Input: part model. Units: mm. Frame: model coordinates. Coordinates: 2 decimals unless noted, no trailing zeros. Write each loop counter-clockwise with the first axis right and the second up, starting at its lowest first coordinate (ties: lowest second). Pieces come first, ordered by that corner, then holes. Notation, with made-up numbers: (-35, 62.5) - (-16, 62.5) arc R21 ccw to (-16, 95.5) - close; hole circle Ø4 at (22.25, -7). An arc over 180 degrees is marked (long way). Use a Markdown table: item, result. Add a question column.
Q1. Section query A-A (z = 0). Return the cut outline in (x, y) (1 decimal), then the cut area to 3 significant figures.
Q2. Material intervals for probe 1 along Z at (x, y) = (-28, 0) (1 decimal); probe 2 along X at (y, z) = (-1.25, 6.25), sorted ascending. Write a range as from..to.
Q3. Pin query (flat end, axial travel): P1, Ø8, axis at x = 156.5, z = 3, coming from the -Y side; P2, Ø6, axis at x = -359, z = -6, coming from the +Y side; P3, Ø2, axis at y = -5, z = -5.5, coming from the -X side; P4, Ø2, axis at x = -271, y = -4.5, coming from the +Z side. Return the tip coordinate at first contact, or that it passes through.
from build123d import *

# Parameters (mm, degrees)
SKETCH_1_R        = 7.9375
SKETCH_1_R_2      = 3.975
EXTRUDE_1_DEPTH   = 493.649
FILLET_1_R        = 2.5
MOVE_BODY_1_ANGLE = 90


with BuildPart() as part:
    # 스케치1 → 보스-돌출1 (new body, symmetric)
    with BuildSketch(Plane(origin=(0, 0, 0), x_dir=(1, 0, 0), z_dir=(0, 1, 0))):
        Circle(SKETCH_1_R)
        Circle(SKETCH_1_R_2, mode=Mode.SUBTRACT)
    extrude(amount=EXTRUDE_1_DEPTH, both=True)

    # 필렛1
    fillet_1_edges = [part.edges().sort_by_distance(p)[0] for p in [
        (-7.9375, -493.649, 0),
        (-7.9375, 493.649, 0),
    ]]
    fillet(fillet_1_edges, radius=FILLET_1_R)


with BuildPart() as part_1:
    # Move Body 1: moved
    add(part.part.rotate(Axis((0, 0, 0), (0, 0, 1)), MOVE_BODY_1_ANGLE))


solid = part_1.part
Values follow:
| question | item | result |
|---|---|---|
| 1 | outline | (-493.6, -5.4) arc R2.5 ccw to (-491.1, -7.9) - (491.1, -7.9) arc R2.5 ccw to (493.6, -5.4) - (493.6, -4) - (-493.6, -4) - close; (-493.6, 4) - (493.6, 4) - (493.6, 5.4) arc R2.5 ccw to (491.1, 7.9) - (-491.1, 7.9) arc R2.5 ccw to (-493.6, 5.4) - close |
| 1 | area | 7,820 mm2 |
| 2 | probe 1 | -7.9..-4, 4..7.9 |
| 2 | probe 2 | -493.47..493.47 |
| 3 | P1 | y = -7.94 |
| 3 | P2 | y = 7.35 |
| 3 | P3 | x = -493.44 |
| 3 | P4 | z = 7.12 |
